Could you check a few things on this drawing? It's one solid part, dimensions in mm from its lowest x, y, z. A direction names the side the tool comes from. Coordinates: 2 decimals unless noted, no trailing zeros. Order: outer loops, then holes, each group sorted by start corner. A loop starts at its lowest first (then second) coordinate and runs counter-clockwise, first axis right, second up. Notation, with made-up numbers: (26, 2) - (62, 2) arc R25 cw to (62, 39) - close; hole circle Ø9 at (88, -8). An arc over 180 degrees is marked (long way). Answer in a Markdown table with one row per item. Add a question column.
Item 1: I want a section at C-C (z = 4). Please give me the cut outline in (x, y) (1 decimal), plus the area to 3 significant figures.
Item 2: I want a section at A-A (x = 7). Please give me the cut outline in (y, z).
Item 3: I want a section at B-B (y = 7). Please give me the cut outline in (x, z).
Item 4: Thinking about a two-plate mould opening in X: for the marked faces 1, 2 and 3, which applies, +X half, -X half, draft (parallel to the pull), parting line (faces both ways), or undercut?
Item 5: If I drill on line 1 along Z through (x, y) = (9.5, 6.5); line 2 along Z through (x, y) = (10, 4); line 3 along X through (y, z) = (24, 3.75), over which ranges is the centre line in solid material (lowest first)? Write a range as from..to.
Item 6: On a 3-axis mill with a long thin cutter (end or side, diameter ignored), from which of +Z, -Z, +X, -X, +Y, -Y can I reach the whole of each face in a straight line? I mean the marked faces 4 and 5. Say none if no direction works.
Item 7: Will these pins go through, and if not, where does the flat tip stop? pin 1 Ø3 at (x, y) = (6, 6) entering from -Z; pin 2 Ø8 at (x, y) = (10, 5) entering from +Z; pin 3 Ø0.5 at (x, y) = (11.5, 12.5) entering from -Z; pin 4 Ø5 at (x, y) = (8, 15.5) entering from +Z.
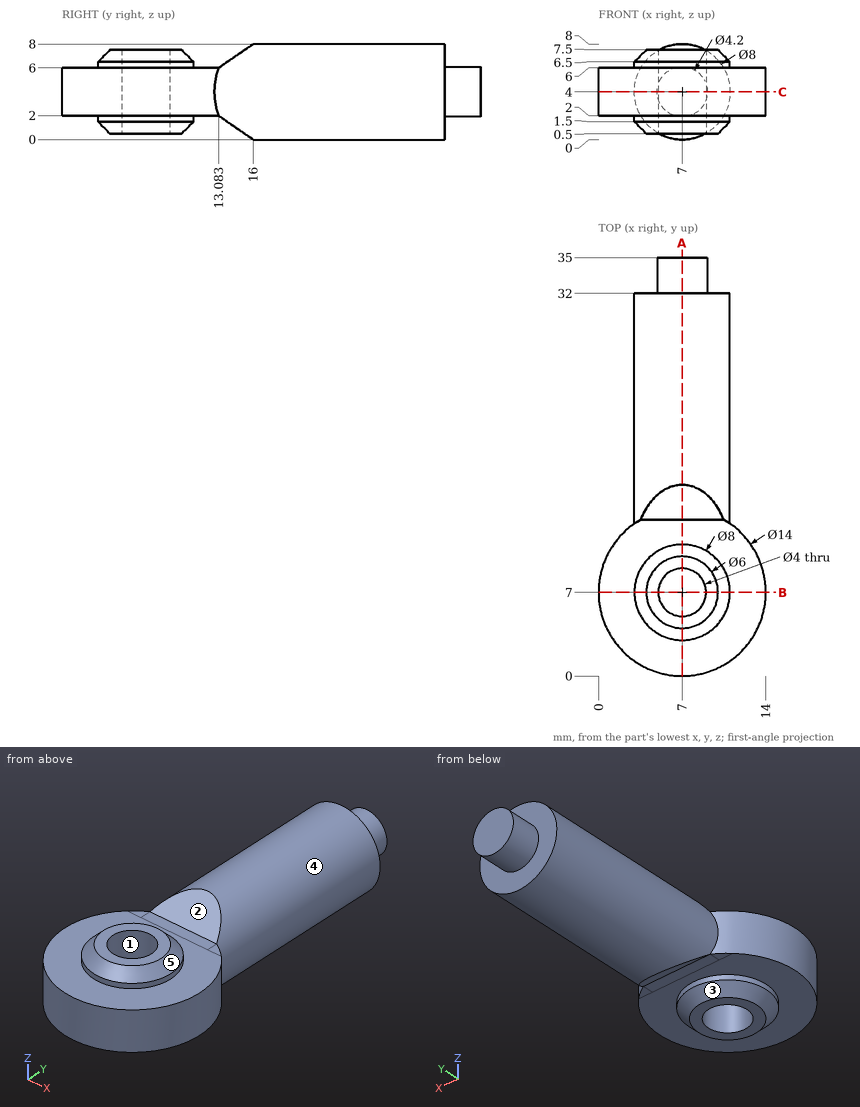
Values follow:
| question | item | result |
|---|---|---|
| 1 | outline | (3, 12.7) arc R7 ccw (long way) to (11, 12.7) - (11, 32) - (9.1, 32) - (9.1, 35) - (4.9, 35) - (4.9, 32) - (3, 32) - close; hole circle Ø4 at (7, 7) |
| 1 | area | 301 mm^2 |
| 2 | outline | (0, 2) - (3, 2) - (3, 1.5) - (4, 0.5) - (5, 0.5) - (5, 7.5) - (4, 7.5) - (3, 6.5) - (3, 6) - (0, 6) - close; (9, 0.5) - (10, 0.5) - (11, 1.5) - (11, 2) - (13.08, 2) - (16, 0) - (32, 0) - (32, 1.9) - (35, 1.9) - (35, 6.1) - (32, 6.1) - (32, 8) - (16, 8) - (13.08, 6) - (11, 6) - (11, 6.5) - (10, 7.5) - (9, 7.5) - close |
| 3 | outline | (0, 2) - (3, 2) - (3, 1.5) - (4, 0.5) - (5, 0.5) - (5, 7.5) - (4, 7.5) - (3, 6.5) - (3, 6) - (0, 6) - close; (9, 0.5) - (10, 0.5) - (11, 1.5) - (11, 2) - (14, 2) - (14, 6) - (11, 6) - (11, 6.5) - (10, 7.5) - (9, 7.5) - close |
| 4 | face 1 | undercut |
| 4 | face 2 | draft |
| 4 | face 3 | parting line |
| 5 | line 1 | z = 0.5..7.5 |
| 5 | line 2 | z = 2..6 |
| 5 | line 3 | x = 3.01..10.99 |
| 6 | face 4 | +Y |
| 6 | face 5 | +Z |
| 7 | pin 1 | stops at z = 0.5 |
| 7 | pin 2 | stops at z = 7.5 |
| 7 | pin 3 | stops at z = 2 |
| 7 | pin 4 | stops at z = 8 |
